Study the drawing (mm; zero at the part's minimum x, y, z) and answer. Round coordinates to 2 decimals unless told otherwise and drop trailing zeros. Loops run counter-clockwise (first coordinate to the right, second up) from the corner with the lowest first, then second, coordinate; pieces in that order, holes last. Notation, with made-up numbers: (39, 17.25) -> (78, 17.25) arc R20 cw to (78, 47.25) -> close; hole circle Ø4 at (38, 12.25). An arc over 180 degrees is marked (long way). Write each question's results on one line, items separated by ' | '. Start each with the question number.
(1) The part is cut by section C-C (y = 34). Determine the outline of the cut face in (x, z), plus the area to 3 significant figures.
(2) The part is cut by section A-A (x = 2.25). Determine the outline of the cut face in (y, z).
(3) Flat-ended cylindrical pins translate along their axes: pin 1 (2.5 mm diameter, centred on x = 2.5, z = 3.5, fed in from +Y); pin 2 (2.5 mm diameter, centred on y = 179.5, z = 2.5, fed in from -X); pin 3 (1.6 mm diameter, centred on x = 2.5, z = 3, fed in from -Y). Find the tip coordinate at first contact, or state that the pin passes through.
(4) The part is cut by section B-B (z = 4.25). Determine the outline of the cut face in (x, y), plus the area to 3 significant figures.
(5) Straight lines are drawn through the part: probe 1 along Y at (x, z) = (1, 2.9); probe 2 along X at (y, z) = (103, 1); probe 3 along Y at (x, z) = (11, 4.2). For each, find the intervals that lie inside material, in ascending order.
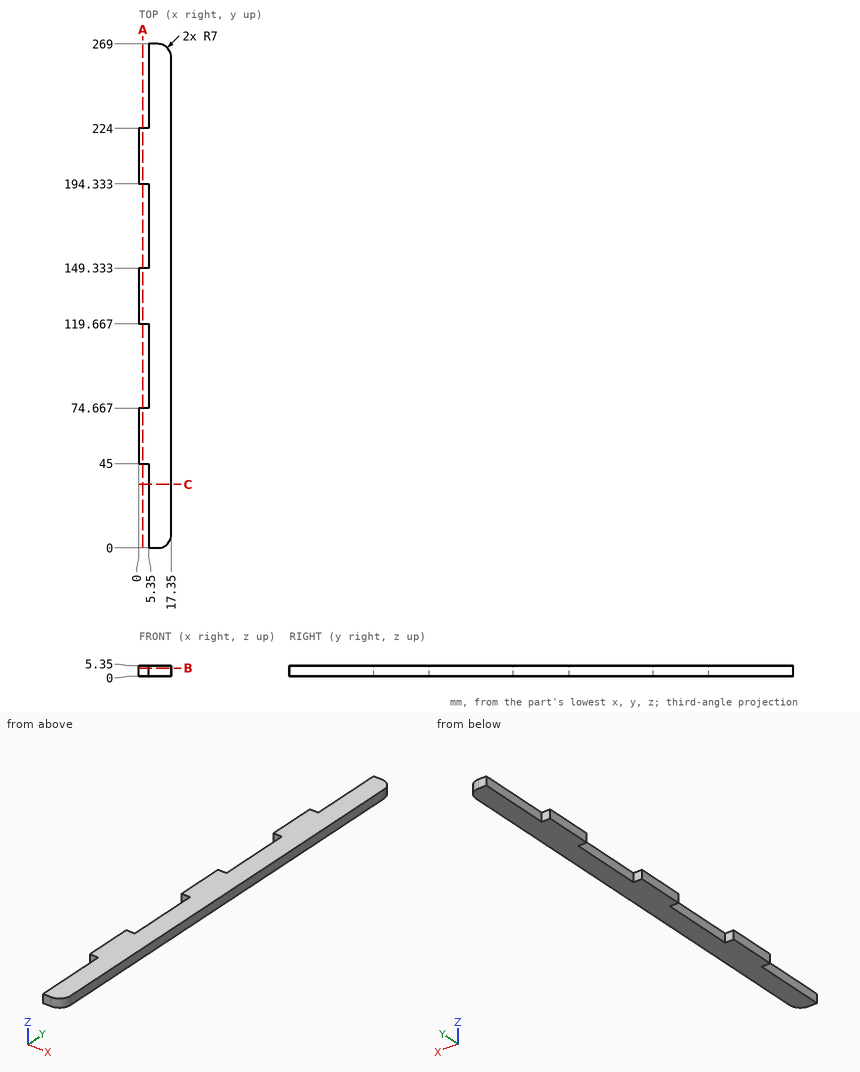
Checked values:
1) outline: (5.35, 0) -> (17.35, 0) -> (17.35, 5.35) -> (5.35, 5.35) -> close | area: 64.2 mm2
2) outline: (45, 0) -> (74.67, 0) -> (74.67, 5.35) -> (45, 5.35) -> close; (119.67, 0) -> (149.33, 0) -> (149.33, 5.35) -> (119.67, 5.35) -> close; (194.33, 0) -> (224, 0) -> (224, 5.35) -> (194.33, 5.35) -> close
3) pin 1: stops at y = 224 | pin 2: stops at x = 5.35 | pin 3: stops at y = 45
4) outline: (0, 45) -> (5.35, 45) -> (5.35, 0) -> (10.35, 0) arc R7 ccw to (17.35, 7) -> (17.35, 262) arc R7 ccw to (10.35, 269) -> (5.35, 269) -> (5.35, 224) -> (0, 224) -> (0, 194.33) -> (5.35, 194.33) -> (5.35, 149.33) -> (0, 149.33) -> (0, 119.67) -> (5.35, 119.67) -> (5.35, 74.67) -> (0, 74.67) -> close | area: 3,680 mm2
5) probe 1: y = 45 to 74.67, 119.67 to 149.33, 194.33 to 224 | probe 2: x = 5.35 to 17.35 | probe 3: y = 0.03 to 268.97
